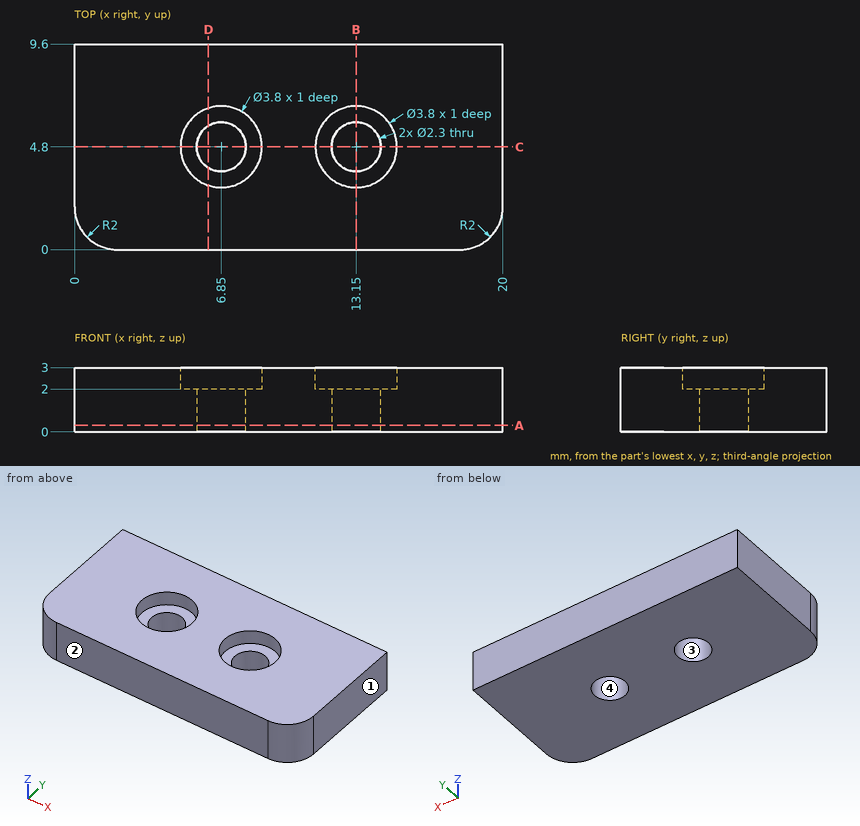
Answer from the drawing. Dimensions are ordinates in mm from the lowest x, y and z of the part. Give positions to 0.01 mm unless a question says otherwise; leave off trailing zeros. Order: outer loops, then holes, each group sorted by start corner. A loop starts at its lowest first (then second) coordinate and runs counter-clockwise, first axis right, second up. Notation, with made-up numbers: (64, 43.25) - (86, 43.25) arc R20 cw to (86, 55.25) - close; hole circle Ø7 at (39.5, 86.25). An arc over 180 degrees is marked (long way). Use one line per item in the form item = value.
1) Find section A-A on z = 0.3. Determine the outline of the cut face in (x, y).
Verdict:
outline = (0, 2) arc R2 ccw to (2, 0) - (18, 0) arc R2 ccw to (20, 2) - (20, 9.6) - (0, 9.6) - close; hole circle Ø2.3 at (6.85, 4.8); hole circle Ø2.3 at (13.15, 4.8)
2) Find section B-B on x = 13.15. Determine the outline of the cut face in (y, z).
Verdict:
outline = (0, 0) - (3.65, 0) - (3.65, 2) - (2.9, 2) - (2.9, 3) - (0, 3) - close; (5.95, 0) - (9.6, 0) - (9.6, 3) - (6.7, 3) - (6.7, 2) - (5.95, 2) - close
3) Find section C-C on y = 4.8. Determine the outline of the cut face in (x, z).
Verdict:
outline = (0, 0) - (5.7, 0) - (5.7, 2) - (4.95, 2) - (4.95, 3) - (0, 3) - close; (8, 0) - (12, 0) - (12, 2) - (11.25, 2) - (11.25, 3) - (8.75, 3) - (8.75, 2) - (8, 2) - close; (14.3, 0) - (20, 0) - (20, 3) - (15.05, 3) - (15.05, 2) - (14.3, 2) - close
4) Find section D-D on x = 6.25. Determine the outline of the cut face in (y, z), and give its area (3 significant figures).
Verdict:
outline = (0, 0) - (3.82, 0) - (3.82, 2) - (3, 2) - (3, 3) - (0, 3) - close; (5.78, 0) - (9.6, 0) - (9.6, 3) - (6.6, 3) - (6.6, 2) - (5.78, 2) - close
area = 21.3 mm^2
5) The mould has two halves that part along X. Classify the marked faces 1, 2, 3 and 4: released by +X, released by -X, zero draft, split by the parting line, or undercut.
Verdict:
face_1 = released by +X
face_2 = zero draft
face_3 = undercut
face_4 = undercut
6) Consider probe 1 along Y at (x, z) = (13.15, 0.95); probe 2 along X at (y, z) = (4.25, 2.1); probe 3 along Y at (x, z) = (13.15, 2.7). Determine where each line is inside the solid, lowest interval first. Write a range as [from, to].
Verdict:
probe_1 = [0, 3.65], [5.95, 9.6]
probe_2 = [0, 5.03], [8.67, 11.33], [14.97, 20]
probe_3 = [0, 2.9], [6.7, 9.6]
7) This flat-tipped pin is pushed along its axis until it touches: pin 1 (1.9 mm diameter, centred on x = 6.5, y = 5.5, fed in from +Z). Where does it stop, or does it pass through?
Verdict:
pin_1 = 2
